Geometry check sheet. Reference: the model listing, model coordinates, mm. A direction names the side the tool comes from. Give positions to 0.01 mm unless a question says otherwise; leave off trailing zeros. Order: outer loops, then holes, each group sorted by start corner. A loop starts at its lowest first (then second) coordinate and runs counter-clockwise, first axis right, second up. Notation, with made-up numbers: M 11.5,55.25 L 46.5,55.25 A17 ccw 46.5,82.25 Z; hole C 38,1.5 d1. An arc over 180 degrees is marked long. Answer as CSV lines item,"result".
Autodesk Inventor part; units mm, degrees
ref_plane "YZ Plane" through (0, 0, 0) normal (1, 0, 0) x (0, 1, 0)
ref_plane "XZ Plane" through (0, 0, 0) normal (0, 1, 0) x (-1, 0, 0)
ref_plane "XY Plane" through (0, 0, 0) normal (0, 0, 1) x (1, 0, 0)
sketch "Sketch1" plane through (0, 0, 0) normal (1, 0, 0) x (0, 1, 0)
  line L0 (35.3248, 26.5797) -> (35.3248, -27.2683)
  line L1 (35.3248, -27.2683) -> (-15.4752, -27.2683)
  line L2 (-15.4752, -27.2683) -> (-15.4752, -14.5683)
  line L3 (-15.4752, -14.5683) -> (-27.319, -14.5683)
  line L4 (-27.319, -14.5683) -> (-27.319, 13.8797)
  line L5 (-27.319, 13.8797) -> (-15.4752, 13.8797)
  line L6 (-15.4752, 13.8797) -> (-15.4752, 26.5797)
  line L7 (-15.4752, 26.5797) -> (35.3248, 26.5797)
  line L8 (-27.319, -0.3443) -> (-33.7293, -0.3443)
  circle A0 centre (32.1498, 23.4047) radius 1.524
  circle A1 centre (32.1498, -24.0933) radius 1.524
  circle A2 centre (-24.144, -10.7583) radius 1.524
  circle A3 centre (-24.144, 10.0697) radius 1.524
  point P0 (0, 0)
  dimension "d0" = 53.848
  dimension "d1" = 12.7
  dimension "d2" = 12.7
  dimension "d3" = 26.924
  dimension "d4" = 50.8
  dimension "d5" = 3.048
  dimension "d6" = 3.048
  dimension "d7" = 3.048
  dimension "d8" = 3.048
  dimension "d9" = 3.175
  dimension "d10" = 3.175
  dimension "d11" = 3.175
  dimension "d12" = 3.175
  dimension "d13" = 16.51
  dimension "d14" = 16.51
  dimension "d15" = 3.175
  dimension "d16" = 3.175
extrude "Extrusion1" add sketch "Sketch1" along normal blind 2.54
properties part number "pixy"
(1) Draft check along Y on faces 1 (the face through (1, 10, 26.58)), 2 (the face through (1, 35.325, 0)), 3 (the face through (1.252, 33.603, 22.947)). Enter one of: +Y half, -Y half, draft (parallel to the pull), parting line (faces both ways), or undercut.
The answers:
face 1,"draft"
face 2,"+Y half"
face 3,"undercut"
(2) Section check A-A on x = 2. Enter the section's corners in (y, z).
The answers:
outline,"M -27.32,-14.57 L -15.48,-14.57 L -15.48,-27.27 L 35.32,-27.27 L 35.32,26.58 L -15.48,26.58 L -15.48,13.88 L -27.32,13.88 Z; hole C -24.14,-10.76 d3.05; hole C -24.14,10.07 d3.05; hole C 32.15,-24.09 d3.05; hole C 32.15,23.4 d3.05"
(3) Tool access check on faces 4 (the face through (1, 10, -27.268)), 5 (the face through (1, -21, -14.568)), 6 (the face through (1, -21, 13.88)). Record the directions out of +Z, -Z, +X, -X, +Y, -Y that give a thin tool (end or side, any length) a straight path to the whole face; none if there is none.
The answers:
face 4,"-Z, +X, -X, +Y, -Y"
face 5,"-Z, +X, -X, -Y"
face 6,"+Z, +X, -X, -Y"
(4) Gauge pin test, flat ends, axial feed: P1, Ø2.5, axis at y = 32.15, z = -24.09, coming from the +X side; P2, Ø1.3, axis at x = 1.5, z = -19.5, coming from the -Y side; P3, Ø5, axis at y = -24.14, z = 10.07, coming from the -X side. Record the tip position at first contact, or that the pin passes through.
The answers:
P1,"passes through"
P2,"stops at y = -15.48"
P3,"stops at x = 0"
(5) Material ranges on line 1 (Z direction, x = 2.2, y = 32); line 2 (Z direction, x = 1.55, y = -23); line 3 (Y direction, x = 1.3, z = 14.5), recorded low to high.
The answers:
line 1,"z = -27.27 to -25.61, -22.58 to 21.89, 24.92 to 26.58"
line 2,"z = -14.57 to -11.77, -9.75 to 9.06, 11.08 to 13.88"
line 3,"y = -15.48 to 35.32"
(6) Section check B-B on z = 15. Enter the section's corners in (x, y), then the cut area to 3 significant figures.
The answers:
outline,"M 0,-15.48 L 2.54,-15.48 L 2.54,35.32 L 0,35.32 Z"
area,"129 mm2"
